Could you check a few things on this model? Use its own coordinates, in mm. Face numbers are marked on the shaded views. A direction names the side the tool comes from. Coordinates: 2 decimals unless noted, no trailing zeros. Loops run counter-clockwise (first coordinate to the right, second up) from the corner with the lowest first, then second, coordinate; pieces in that order, holes last.
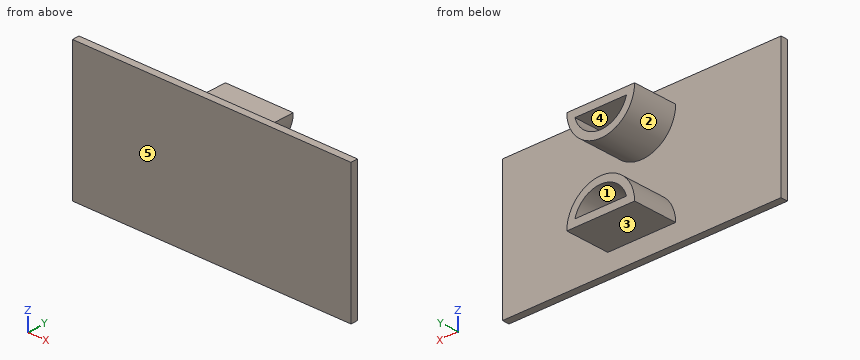
from build123d import *

# Parameters (mm, degrees)
SKETCH1_W           = 39
SKETCH1_H           = 19
BOSS_EXTRUDE1_DEPTH = 1
BOSS_EXTRUDE2_DEPTH = 6.25


with BuildPart() as part:
    # Sketch1 → Boss-Extrude1 (new body)
    with BuildSketch(Plane(origin=(0, 0, 0), x_dir=(1, 0, 0), z_dir=(0, 1, 0))):
        with Locations((7.081578947, 0.711842105)):
            Rectangle(SKETCH1_W, SKETCH1_H)
    extrude(amount=BOSS_EXTRUDE1_DEPTH)

    # Sketch2 → Boss-Extrude2 (add)
    # profile 1 of 2: a face of its own
    with BuildSketch(Plane(origin=(0, 1, 0), x_dir=(1, 0, 0), z_dir=(0, 1, 0))):
        with BuildLine():
            Line((2.331578947, 7.661842105), (11.831578947, 7.661842105))
            ThreePointArc((11.831578947, 7.661842105), (7.081578947, 2.911842105), (2.331578947, 7.661842105))
        make_face()
        with BuildLine():
            Line((3.467370874, 6.661842105), (10.695787021, 6.661842105))
            ThreePointArc((10.695787021, 6.661842105), (7.081578947, 3.911842105), (3.467370874, 6.661842105))
        make_face(mode=Mode.SUBTRACT)
    # profile 2 of 2: a face of its own
    with BuildSketch(Plane(origin=(0, 1, 0), x_dir=(1, 0, 0), z_dir=(0, 1, 0))):
        with BuildLine():
            Line((2.331578947, -6.238157895), (11.831578947, -6.238157895))
            ThreePointArc((11.831578947, -6.238157895), (7.081578947, -1.488157895), (2.331578947, -6.238157895))
        make_face()
        with BuildLine():
            Line((3.467370874, -5.238157895), (10.695787021, -5.238157895))
            ThreePointArc((10.695787021, -5.238157895), (7.081578947, -2.488157895), (3.467370874, -5.238157895))
        make_face(mode=Mode.SUBTRACT)
    extrude(amount=BOSS_EXTRUDE2_DEPTH)


solid = part.part
(1) Imagine slicing it at B-B, the plane x = 4.5. Write out the boundary of the cut face in (y, z), and give its area (3 significant figures).
Answers:
outline: (0, -10.21) - (1, -10.21) - (1, -7.66) - (7.25, -7.66) - (7.25, -6.66) - (1, -6.66) - (1, -4.94) - (7.25, -4.94) - (7.25, -3.67) - (1, -3.67) - (1, 2.25) - (7.25, 2.25) - (7.25, 3.52) - (1, 3.52) - (1, 5.24) - (7.25, 5.24) - (7.25, 6.24) - (1, 6.24) - (1, 8.79) - (0, 8.79) - close
area: 47.3 mm2
(2) Imagine slicing it at D-D, the plane x = -5.5. Write out the boundary of the cut face in (y, z).
Answers:
outline: (0, -10.21) - (1, -10.21) - (1, 8.79) - (0, 8.79) - close
(3) We'd pull the mould along X, two halves only. Please class the marked faces 1, 2 and 3: +X half, -X half, draft (parallel to the pull), parting line (faces both ways), or undercut.
Answers:
face 1: undercut
face 2: parting line
face 3: draft
(4) Imagine slicing it at C-C, the plane z = 3. Write out the boundary of the cut face in (x, y).
Answers:
outline: (-12.42, 0) - (26.58, 0) - (26.58, 1) - (10.56, 1) - (10.56, 7.25) - (8.97, 7.25) - (8.97, 1) - (5.19, 1) - (5.19, 7.25) - (3.61, 7.25) - (3.61, 1) - (-12.42, 1) - close
(5) For pin 1 (5.5 mm diameter, centred on x = 12, z = -1.5, fed in from +Y); pin 2 (3 mm diameter, centred on x = 6.5, y = 5.5, fed in from +Z), each with a flat end and sliding along its axis, tell me the tip position at first contact or that it passes through.
Answers:
pin 1: stops at y = 1
pin 2: stops at z = 6.24
(6) Imagine slicing it at A-A, the plane y = 1.75. Write out the boundary of the cut face in (x, z), and give its area (3 significant figures).
Answers:
outline: (2.33, -7.66) - (11.83, -7.66) arc R4.75 ccw to start; (2.33, 6.24) arc R4.75 ccw to (11.83, 6.24) - close; hole (3.47, -6.66) - (10.7, -6.66) arc R3.75 ccw to start; hole (3.47, 5.24) arc R3.75 ccw to (10.7, 5.24) - close
area: 41.5 mm2
(7) Which directions (+Z, -Z, +X, -X, +Y, -Y) give clear straight access to the entire face, cutting with the end or side of a thin tool? Please do the marked faces 4 and 5.
Answers:
face 4: +Y
face 5: +Z, -Z, +X, -X, -Y
(8) I need wall thicknesses on probe 1 along Z at (x, y) = (8, 5.5); probe 2 along Z at (x, y) = (5, 2); probe 3 along Y at (x, z) = (21, 3.5). Which ranges of each line are inside material? Lowest first, please.
Answers:
probe 1: z = -7.66 to -6.66, -4.03 to -3, 1.58 to 2.6, 5.24 to 6.24
probe 2: z = -7.66 to -6.66, -4.54 to -3.39, 1.97 to 3.12, 5.24 to 6.24
probe 3: y = 0 to 1
